The figure shows three views and two pictorial views of one solid part (mm, origin at its lowest corner). Answer the questions. A direction names the side the tool comes from. Round coordinates to 2 decimals unless told otherwise and drop trailing zeros. Order: outer loops, then holes, each group sorted by start corner. A loop starts at its lowest first (then second) coordinate and runs counter-clockwise, first axis right, second up. Notation, with made-up numbers: (-17.75, 18.5) - (1.25, 18.5) arc R29 ccw to (1.25, 55.5) - close; hole circle Ø5 at (-38.5, 66). An arc over 180 degrees is marked (long way). Answer as a JSON object with one key per item and string values. Group by question number.
Q1. Given pin 1 Ø11.5 at (x, z) = (231.78, 369.43) entering from -Y; pin 2 Ø6 at (x, y) = (180, 225) entering from -Z; pin 3 Ø2 at (x, z) = (271, 400) entering from +Y, each flat-ended and moving along its own axis, determine where each tip first touches the part or whether it passes through.
Q2. Consider line 1 (X direction, y = 129, z = 305.5); line 2 (Z direction, x = 121.5, y = 141.5); line 3 (Y direction, x = 176.5, z = 236). Determine where each line is inside the solid, lowest interval first.
Q3. A tool of negligible diameter and unlimited length cuts with its end or side. For the marked faces 4 and 5, from which of +Z, -Z, +X, -X, +Y, -Y can it reach the whole face along a straight path? Write none if from no direction.
Q4. A cutting plane is placed at C-C on z = 335.5. Determine the outline of the cut face in (x, y), and give its area (3 significant figures).
Q5. A cutting plane is placed at B-B on x = 59.5. Determine the outline of the cut face in (y, z), and give its area (3 significant figures).
Q6. The mould has two halves that part along Z. Classify the marked faces 1, 2 and 3: pulls with the +Z half, pulls with the -Z half, needs draft (parallel to the pull), parting line crosses it, or undercut.
Q7. A cutting plane is placed at A-A on y = 195.5. Determine the outline of the cut face in (x, z).
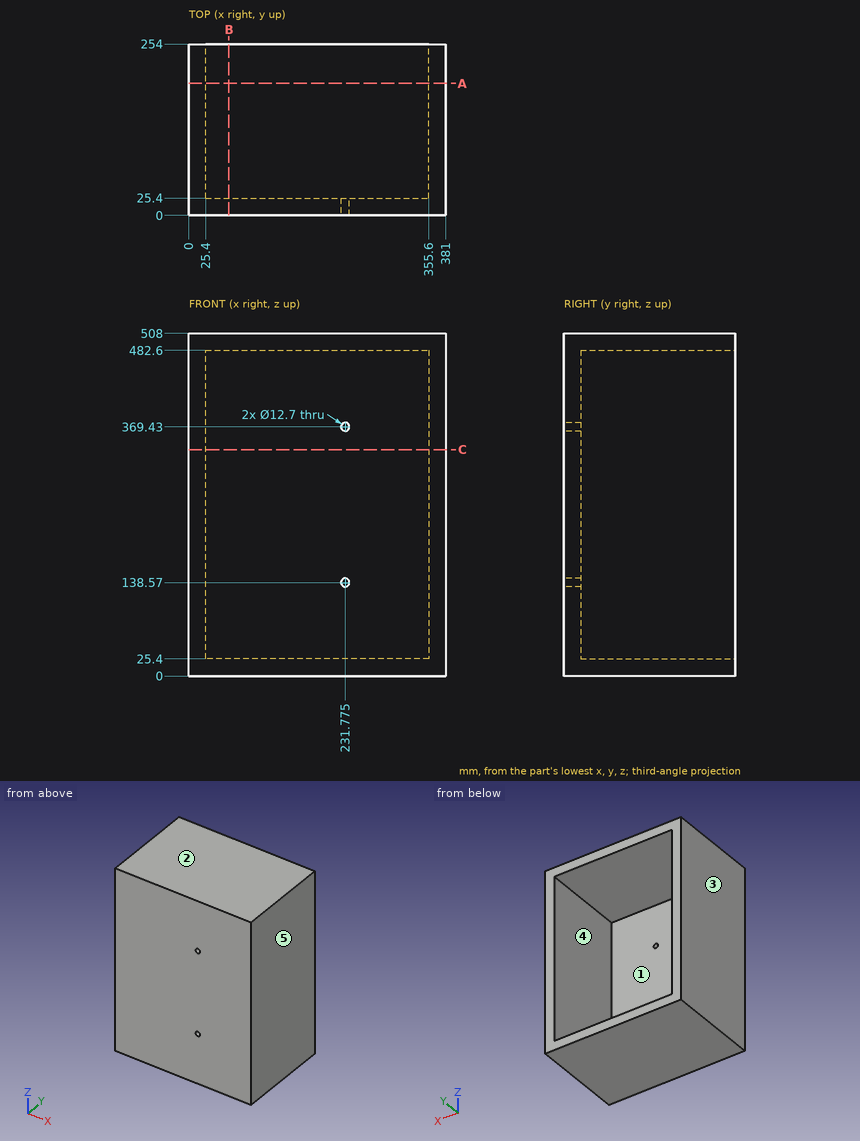
Result set:
{
 "1": {"pin 1": "passes through", "pin 2": "stops at z = 0", "pin 3": "stops at y = 25.4"},
 "2": {"line 1": "x = 0 to 25.4, 355.6 to 381", "line 2": "z = 0 to 25.4, 482.6 to 508", "line 3": "y = 0 to 25.4"},
 "3": {"face 4": "+Y", "face 5": "+Z, -Z, +X, +Y, -Y"},
 "4": {"outline": "(0, 0) - (381, 0) - (381, 254) - (355.6, 254) - (355.6, 25.4) - (25.4, 25.4) - (25.4, 254) - (0, 254) - close", "area": "21,300 mm²"},
 "5": {"outline": "(0, 0) - (254, 0) - (254, 25.4) - (25.4, 25.4) - (25.4, 482.6) - (254, 482.6) - (254, 508) - (0, 508) - close", "area": "24,500 mm²"},
 "6": {"face 1": "undercut", "face 2": "pulls with the +Z half", "face 3": "needs draft"},
 "7": {"outline": "(0, 0) - (381, 0) - (381, 508) - (0, 508) - close; hole (25.4, 25.4) - (355.6, 25.4) - (355.6, 482.6) - (25.4, 482.6) - close"}
}
